Geometry check sheet. Reference: drawing and pictorial views, mm from the part's lowest x, y, z. A direction names the side the tool comes from. Round coordinates to 2 decimals unless told otherwise and drop trailing zeros. Use one line per item in the form item = value.
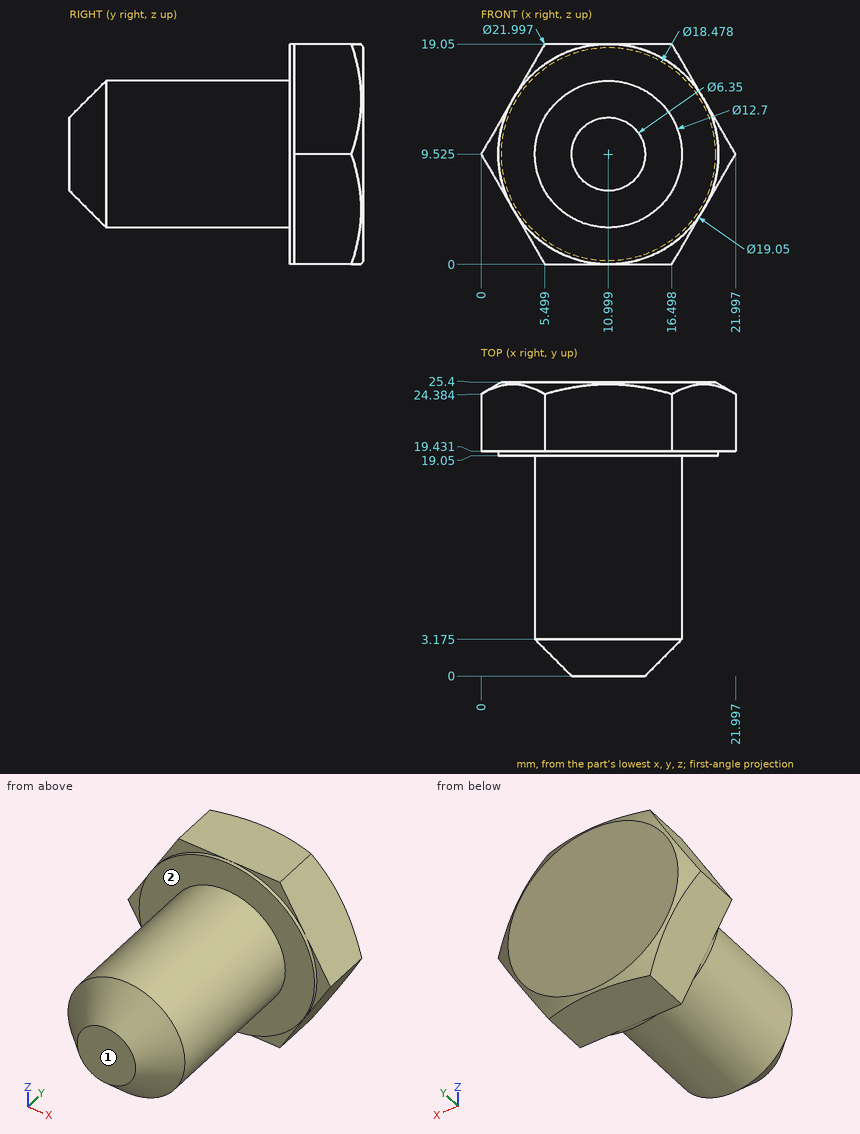
1. Gauge pin test, flat ends, axial feed: pin 1 (2 mm diameter, centred on y = 17.5, z = 13, fed in from -X); pin 2 (4 mm diameter, centred on x = 18, z = 16, fed in from +Y); pin 3 (8 mm diameter, centred on y = 20.5, z = 2, fed in from -X) (1 decimal); pin 4 (2 mm diameter, centred on x = 6, y = 5.5, fed in from +Z). Record the tip position at first contact, or that the pin passes through.
Return value:
pin_1 = 5.15
pin_2 = 25.4
pin_3 = 2
pin_4 = 14.46
2. Material ranges on line 1 along Y through (x, z) = (5.5, 4.5); line 2 along X through (y, z) = (10.25, 9.75) (1 decimal); line 3 along Y through (x, z) = (6.5, 7.5), recorded low to high.
Return value:
line_1 = 19.05 to 25.4
line_2 = 4.7 to 17.3
line_3 = 1.76 to 25.4
3. Tool access check on the marked faces 1 and 2. Record the directions out of +Z, -Z, +X, -X, +Y, -Y that give a thin tool (end or side, any length) a straight path to the whole face; none if there is none.
Return value:
face_1 = +Z, -Z, +X, -X, -Y
face_2 = -Y
